Could you check a few things on this model? Use its own coordinates, in mm. A direction names the side the tool comes from. Round coordinates to 2 decimals unless told otherwise and drop trailing zeros. Order: outer loops, then holes, each group sorted by start corner. A loop starts at its lowest first (then second) coordinate and runs counter-clockwise, first axis right, second up. Notation, with made-up numbers: (5.5, 55.5) -> (61.5, 55.5) arc R16 cw to (61.5, 79.5) -> close; hole circle Ø9 at (34, 27). An arc over 180 degrees is marked (long way). One line per question, with ' | ' between items.
```python
from build123d import *

# Parameters (mm, degrees)
F0_W     = 50.8
F0_H     = 38.1
F1_DEPTH = 31.75
F2_W     = 25.4
F2_H     = 19.05
F3_DEPTH = 12.7
F5_DEPTH = 50.8


with BuildPart() as f1:
    # F0 (on Front) → F1 (new body)
    with BuildSketch(Plane.XZ):
        with Locations((25.4, 19.05)):
            Rectangle(F0_W, F0_H)
    extrude(amount=F1_DEPTH)

    # F2 (on face) → F3 (cut)
    with BuildSketch(Plane(origin=(0, 0, 0), x_dir=(-1, 0, 0), z_dir=(0, 1, 0))):
        with Locations((-25.4, 28.575)):
            Rectangle(F2_W, F2_H)
    extrude(amount=-F3_DEPTH, mode=Mode.SUBTRACT)

    # F4 (on face) → F5 (cut)
    with BuildSketch(Plane.YZ.offset(50.8)):
        with BuildLine():
            Line((-31.75, 38.1), (-6.35, 38.1))
            ThreePointArc((-6.35, 38.1), (-49.710512, 56.060512), (-31.75, 12.7))
            Line((-31.75, 12.7), (-31.75, 38.1))
        make_face()
        with BuildLine():
            ThreePointArc((-31.75, 12.7), (-13.789488, 20.139488), (-6.35, 38.1))
            Line((-6.35, 38.1), (-31.75, 38.1))
            Line((-31.75, 38.1), (-31.75, 12.7))
        make_face()
    extrude(amount=-F5_DEPTH, mode=Mode.SUBTRACT)


solid = f1.part
```
1. I want a section at B-B on z = 22.5. List the corners of the cut face in (x, y) for me, and give its area (3 significant figures).
From the geometry:
outline: (0, -11.71) -> (12.7, -11.71) -> (12.7, 0) -> (0, 0) -> close; (38.1, -11.71) -> (50.8, -11.71) -> (50.8, 0) -> (38.1, 0) -> close | area: 297 mm²
2. I need wall thicknesses on probe 1 along X at (y, z) = (-7, 24); probe 2 along Z at (x, y) = (14.5, -6); probe 3 along Y at (x, z) = (8, 15). Which ranges of each line are inside material? Lowest first, please.
From the geometry:
probe 1: x = 0 to 12.7, 38.1 to 50.8 | probe 2: z = 0 to 19.05 | probe 3: y = -21.19 to 0
3. I want a section at C-C on y = -4. List the corners of the cut face in (x, z) for me, and give its area (3 significant figures).
From the geometry:
outline: (0, 0) -> (50.8, 0) -> (50.8, 38.1) -> (38.1, 38.1) -> (38.1, 19.05) -> (12.7, 19.05) -> (12.7, 38.1) -> (0, 38.1) -> close | area: 1,450 mm²
4. On a 3-axis mill with a long thin cutter (end or side, diameter ignored), from which of +Z, -Z, +X, -X, +Y, -Y can I reach the whole of each face in a straight line? I mean faces 4 (the face through (6, -3, 38.1)), 5 (the face through (26, -6, 19.05)). Say none if no direction works.
From the geometry:
face 4: +Z, +X, -X, +Y, -Y | face 5: +Z, +Y
5. I want a section at A-A on x = 26.5. List the corners of the cut face in (y, z) for me.
From the geometry:
outline: (-31.75, 0) -> (0, 0) -> (0, 19.05) -> (-12.7, 19.05) -> (-12.7, 21.3) arc R25.4 cw to (-31.75, 12.7) -> close
6. If we mould it in two halves opening along X, with no side actions, what happens to faces 1 (the face through (0, -12, 15)), 2 (the face through (26, -12.7, 20)), 3 (the face through (50.8, -12, 15))? For each: pulls with the +X half, pulls with the -X half, needs draft (parallel to the pull), parting line crosses it, or undercut.
From the geometry:
face 1: pulls with the -X half | face 2: undercut | face 3: pulls with the +X half
7. I'm going to push flat-ended pins straight in: pin 1 (8 mm diameter, centred on x = 32.5, y = -18, fed in from +Z); pin 2 (5 mm diameter, centred on x = 19, y = -9.5, fed in from +Z); pin 3 (4 mm diameter, centred on x = 15.5, z = 24, fed in from +Y); pin 4 (0.7 mm diameter, centred on x = 26.5, z = 20.5, fed in from +Y). Where does each tip first touch, or does it pass through?
From the geometry:
pin 1: stops at z = 19.93 | pin 2: stops at z = 19.05 | pin 3: passes through | pin 4: stops at y = -12.7
8. I want a section at D-D on x = 5. List the corners of the cut face in (y, z) for me.
From the geometry:
outline: (-31.75, 0) -> (0, 0) -> (0, 38.1) -> (-6.35, 38.1) arc R25.4 cw to (-31.75, 12.7) -> close
